Could you check a few things on this drawing? It's one solid part, dimensions in mm from its lowest x, y, z. A direction names the side the tool comes from. Round coordinates to 2 decimals unless told otherwise and drop trailing zeros. Write each loop counter-clockwise with the first axis right and the second up, starting at its lowest first coordinate (ties: lowest second). Pieces come first, ordered by that corner, then holes. Notation, with made-up numbers: (73, 67) - (92, 67) arc R15 ccw to (92, 95) - close; hole circle Ø8 at (-22, -9.5). An arc over 180 degrees is marked (long way). Use one line per item in the form item = value. Start each with the question number.
1. Will these pins go through, and if not, where does the flat tip stop? pin 1 (4 mm diameter, centred on x = 19, y = 4, fed in from -Z); pin 2 (14.5 mm diameter, centred on x = 22.5, z = 67.5, fed in from -Y); pin 3 (17 mm diameter, centred on x = 112.5, z = 22.5, fed in from +Y).
2. Which directions (+Z, -Z, +X, -X, +Y, -Y) give clear straight access to the entire face, cutting with the end or side of a thin tool? Please do the marked faces 1 and 2.
3. I want a section at B-B, the plane x = 67.5. List the corners of the cut face in (y, z) for me, plus the area to 3 significant figures.
4. We'd pull the mould along Z, two halves only. Please class the marked faces 3, 4 and 5: +Z half, -Z half, draft (parallel to the pull), parting line (faces both ways), or undercut.
5. If I drill on line 1 along Z through (x, y) = (112.5, 17); line 2 along X through (y, z) = (8, 67.5); line 3 along X through (y, z) = (20, 67.5), over which ranges is the centre line in solid material (lowest first)?
6. I want a section at A-A, the plane z = 67.5. List the corners of the cut face in (x, y) for me.
7. I want a section at C-C, the plane y = 2.5. List the corners of the cut face in (x, z) for me.
8. I want a section at D-D, the plane z = 22.5. List the corners of the cut face in (x, y) for me.
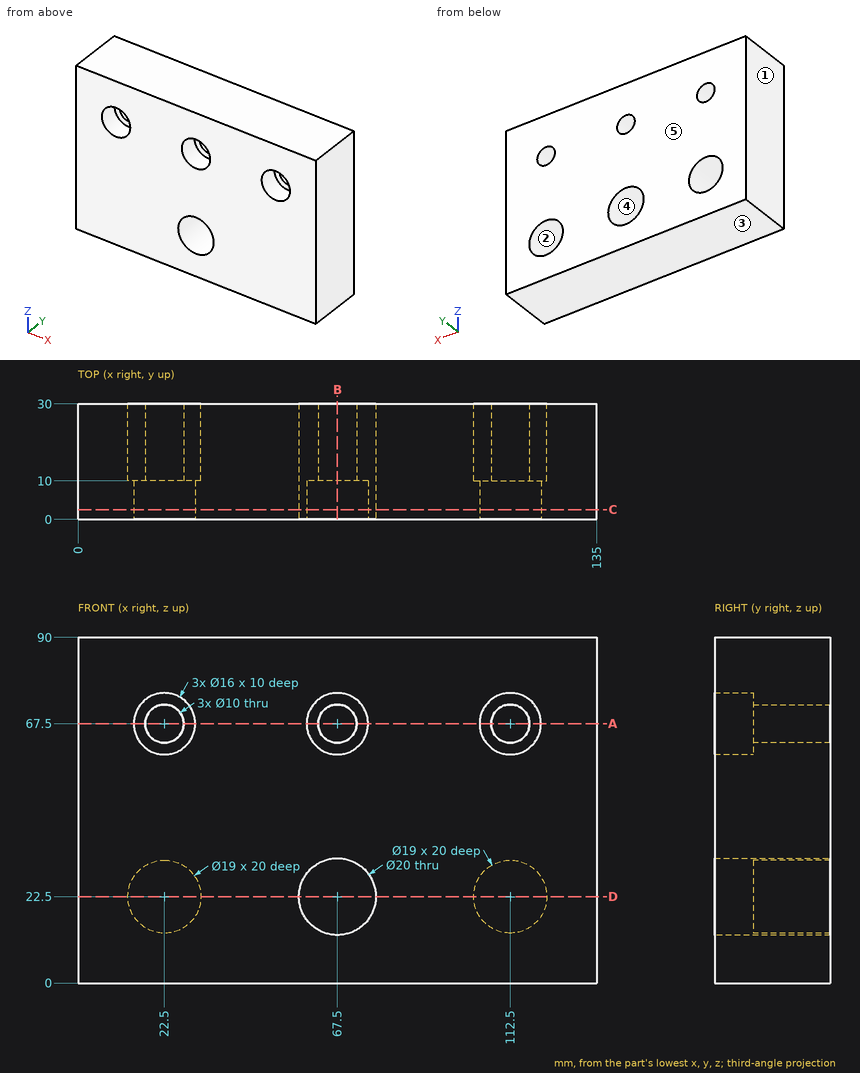
Model answer:
q1.pin_1 = 0
q1.pin_2 = 10
q1.pin_3 = 10
q2.face_1 = +Z, -Z, -X, +Y, -Y
q2.face_2 = +Y
q3.outline = (0, 0) - (30, 0) - (30, 12.5) - (0, 12.5) - close; (0, 32.5) - (30, 32.5) - (30, 62.5) - (10, 62.5) - (10, 59.5) - (0, 59.5) - close; (0, 75.5) - (10, 75.5) - (10, 72.5) - (30, 72.5) - (30, 90) - (0, 90) - close
q3.area = 1,740 mm2
q4.face_3 = -Z half
q4.face_4 = undercut
q4.face_5 = draft
q5.line_1 = 0 to 13, 32 to 62.5, 72.5 to 90
q5.line_2 = 0 to 14.5, 30.5 to 59.5, 75.5 to 104.5, 120.5 to 135
q5.line_3 = 0 to 17.5, 27.5 to 62.5, 72.5 to 107.5, 117.5 to 135
q6.outline = (0, 0) - (14.5, 0) - (14.5, 10) - (17.5, 10) - (17.5, 30) - (0, 30) - close; (27.5, 10) - (30.5, 10) - (30.5, 0) - (59.5, 0) - (59.5, 10) - (62.5, 10) - (62.5, 30) - (27.5, 30) - close; (72.5, 10) - (75.5, 10) - (75.5, 0) - (104.5, 0) - (104.5, 10) - (107.5, 10) - (107.5, 30) - (72.5, 30) - close; (117.5, 10) - (120.5, 10) - (120.5, 0) - (135, 0) - (135, 30) - (117.5, 30) - close
q7.outline = (0, 0) - (135, 0) - (135, 90) - (0, 90) - close; hole circle Ø16 at (22.5, 67.5); hole circle Ø20 at (67.5, 22.5); hole circle Ø16 at (67.5, 67.5); hole circle Ø16 at (112.5, 67.5)
q8.outline = (0, 0) - (57.5, 0) - (57.5, 30) - (32, 30) - (32, 10) - (13, 10) - (13, 30) - (0, 30) - close; (77.5, 0) - (135, 0) - (135, 30) - (122, 30) - (122, 10) - (103, 10) - (103, 30) - (77.5, 30) - close
